Here's how the part is built. I have some questions about the finished solid (model axes, mm). Face numbers are marked on the shaded views. Coordinates: 2 decimals unless noted, no trailing zeros. Loops run counter-clockwise (first coordinate to the right, second up) from the corner with the lowest first, then second, coordinate; pieces in that order, holes last. Notation, with made-up numbers: (-1.75, -13.75) -> (3.25, -13.75) arc R19 ccw to (3.25, -0.75) -> close; hole circle Ø4 at (35, 53.5). An arc over 180 degrees is marked (long way). Answer as a JSON object with one key per item and string values. Group by question number.
1) I need wall thicknesses on probe 1 along Y at (x, z) = (101, 35); probe 2 along X at (y, z) = (50, 25); probe 3 along Y at (x, z) = (99, 18). Which ranges of each line are inside material? Lowest first, please. Write a range as [from, to].
2) I want a section at A-A (x = 101.6). Write out the boundary of the cut face in (y, z), then the cut area to 3 significant figures.
3) I want a section at B-B (y = 50.8). Write out the boundary of the cut face in (x, z).
4) If we mould it in two halves opening along X, with no side actions, what happens to the marked faces 1, 2, 3 and 4? For each: +X half, -X half, draft (parallel to the pull), parting line (faces both ways), or undercut.
5) I want a section at C-C (z = 17.5). Write out the boundary of the cut face in (x, y), then the cut area to 3 significant figures.
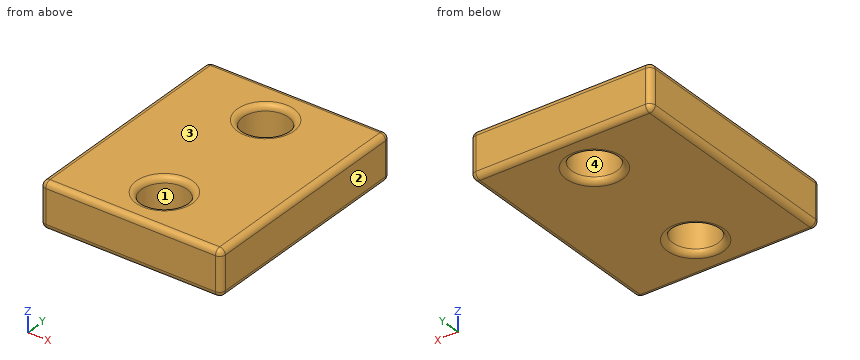
```python
from build123d import *

# Parameters (mm, degrees)
F0_W     = 203.2
F0_H     = 254
F0_R     = 25.4
F1_DEPTH = 50.8
F2_R     = 6.35


with BuildPart() as f1:
    # F0 (on Top) → F1 (new body)
    with BuildSketch(Plane.XY):
        with Locations((101.6, 127)):
            Rectangle(F0_W, F0_H)
        with Locations((101.6, 50.8)):
            Circle(F0_R, mode=Mode.SUBTRACT)
        with Locations((101.6, 203.2)):
            Circle(F0_R, mode=Mode.SUBTRACT)
    extrude(amount=F1_DEPTH)

    # F2
    f2_edges = [f1.edges().sort_by_distance(p)[0] for p in [
        (0, 254, 25.4),
        (0, 0, 25.4),
        (0, 127, 0),
        (0, 127, 50.8),
        (203.2, 254, 25.4),
        (101.6, 254, 0),
        (101.6, 254, 50.8),
        (76.2, 203.2, 50.8),
        (76.2, 50.8, 50.8),
        (127, 50.8, 25.4),
        (76.2, 50.8, 0),
        (127, 203.2, 25.4),
        (76.2, 203.2, 0),
        (203.2, 0, 25.4),
        (101.6, 0, 0),
        (101.6, 0, 50.8),
        (203.2, 127, 0),
        (203.2, 127, 50.8),
    ]]
    fillet(f2_edges, radius=F2_R)


solid = f1.part
```
Determined:
{
 "1": {"probe 1": "[0, 25.41], [76.19, 177.81], [228.59, 254]", "probe 2": "[0, 76.21], [126.99, 203.2]", "probe 3": "[0, 25.53], [76.07, 177.93], [228.47, 254]"},
 "2": {"outline": "(0, 6.35) arc R6.35 ccw to (6.35, 0) -> (19.05, 0) arc R6.35 ccw to (25.4, 6.35) -> (25.4, 44.45) arc R6.35 ccw to (19.05, 50.8) -> (6.35, 50.8) arc R6.35 ccw to (0, 44.45) -> close; (76.2, 6.35) arc R6.35 ccw to (82.55, 0) -> (171.45, 0) arc R6.35 ccw to (177.8, 6.35) -> (177.8, 44.45) arc R6.35 ccw to (171.45, 50.8) -> (82.55, 50.8) arc R6.35 ccw to (76.2, 44.45) -> close; (228.6, 6.35) arc R6.35 ccw to (234.95, 0) -> (247.65, 0) arc R6.35 ccw to (254, 6.35) -> (254, 44.45) arc R6.35 ccw to (247.65, 50.8) -> (234.95, 50.8) arc R6.35 ccw to (228.6, 44.45) -> close", "area": "7,640 mm^2"},
 "3": {"outline": "(0, 6.35) arc R6.35 ccw to (6.35, 0) -> (69.85, 0) arc R6.35 ccw to (76.2, 6.35) -> (76.2, 44.45) arc R6.35 ccw to (69.85, 50.8) -> (6.35, 50.8) arc R6.35 ccw to (0, 44.45) -> close; (127, 6.35) arc R6.35 ccw to (133.35, 0) -> (196.85, 0) arc R6.35 ccw to (203.2, 6.35) -> (203.2, 44.45) arc R6.35 ccw to (196.85, 50.8) -> (133.35, 50.8) arc R6.35 ccw to (127, 44.45) -> close"},
 "4": {"face 1": "undercut", "face 2": "+X half", "face 3": "draft", "face 4": "undercut"},
 "5": {"outline": "(0, 6.35) arc R6.35 ccw to (6.35, 0) -> (196.85, 0) arc R6.35 ccw to (203.2, 6.35) -> (203.2, 247.65) arc R6.35 ccw to (196.85, 254) -> (6.35, 254) arc R6.35 ccw to (0, 247.65) -> close; hole circle Ø50.8 at (101.6, 50.8); hole circle Ø50.8 at (101.6, 203.2)", "area": "47,500 mm^2"}
}
